Part model, mm, in its own coordinate system. A direction names the side the tool comes from. Round coordinates to 2 decimals unless told otherwise and drop trailing zeros. Loops run counter-clockwise (first coordinate to the right, second up) from the corner with the lowest first, then second, coordinate; pieces in that order, holes last.
(1) Tool access for faces 1 (the face through (30, 41, -3)), 2 (the face through (68, 13, -4)), 3 (the face through (50, 23, -3.1)), 4 (the face through (33, 12, -4)): list every direction of +Z, -Z, +X, -X, +Y, -Y with a clear straight run to the whole face (end or side of a thin tool).
(2) Cut at D-D on x = 27. List the corners of the cut face in (y, z).
(3) Mould opens along X. For faces 5 (the face through (70, 41, -3)), 6 (the face through (16.547, 5.382, 1.875)), 7 (the face through (44, 29, 3.5)) say: +X half, -X half, draft (parallel to the pull), parting line (faces both ways), or undercut.
(4) Cut at C-C on z = 1. List the corners of the cut face in (x, y) (3 decimals).
(5) Flat gauge pins, fed straight in: pin 1 (2.5 mm diameter, centred on y = 42, z = -3.5, fed in from +X); pin 2 (2.5 mm diameter, centred on y = 40, z = -3, fed in from -X); pin 3 (0.6 mm diameter, centred on x = 43.5, z = -4, fed in from -Y). Where does each tip first touch, or does it go through?
(6) Cut at A-A on y = 33.5. List the corners of the cut face in (x, z), then the cut area to 3 significant figures.
(7) Probe probe 1 along Y at (x, z) = (15, 2.7); probe 2 along Z at (x, y) = (43, 17); probe 3 along Z at (x, y) = (73.5, 20). List the from-to ranges inside material, lowest first.
(8) Cut at B-B on x = 15. List the corners of the cut face in (y, z), then the cut area to 3 significant figures.
Autodesk Inventor part; units mm, degrees
ref_plane "YZ Plane" through (0, 0, 0) normal (1, 0, 0) x (0, 1, 0)
ref_plane "XZ Plane" through (0, 0, 0) normal (0, 1, 0) x (-1, 0, 0)
ref_plane "XY Plane" through (0, 0, 0) normal (0, 0, 1) x (1, 0, 0)
sketch "Sketch1" plane through (0, 0, 0) normal (0, 0, 1) x (1, 0, 0)
  line L0 (0, 0) -> (90, 0)
  line L1 (90, 0) -> (90, 57)
  line L2 (90, 57) -> (0, 57)
  line L3 (0, 57) -> (0, 0)
  circle A0 centre (15, 53) radius 1.55
  circle A1 centre (15, 4.74) radius 1.55
  circle A2 centre (80.699, 49.825) radius 1.55
  circle A3 centre (80.699, 7.915) radius 1.55
  dimension "d0" = 57
  dimension "d1" = 90
  dimension "d2" = 3.1
  dimension "d3" = 3.1
  dimension "d4" = 3.1
  dimension "d5" = 3.1
  dimension "d6" = 4
  dimension "d7" = 15
  dimension "d8" = 48.26
  dimension "d9" = 15
  dimension "d10" = 80.699
  dimension "d11" = 7.175
  dimension "d12" = 41.91
  dimension "d13" = 80.699
extrude "Extrusion1" add sketch "Sketch1" along normal blind 3.5
sketch "Sketch2" plane through (0, 0, 0) normal (0, 0, -1) x (-1, 0, 0)
  line L0 (-70, 35) -> (-30, 35)
  line L1 (-30, 35) -> (-30, 57)
  line L2 (-30, 57) -> (-70, 57)
  line L3 (-70, 57) -> (-70, 35)
  line L4 (0, 0) -> (-90, 0)
  line L5 (-90, 57) -> (0, 57)
  line L6 (-90, 0) -> (-90, 57)
  dimension "d16" = 35
  dimension "d17" = 40
  dimension "d18" = 20
extrude "Extrusion2" add sketch "Sketch2" along normal blind 5.1
sketch "Sketch3" plane through (30, 35, 0) normal (0, -1, 0) x (1, 0, 0)
  line L0 (0, -5.1) -> (40, -5.1)
  line L1 (40, -5.1) -> (40, -3.1)
  line L2 (40, -3.1) -> (0, -3.1)
  line L3 (0, -3.1) -> (0, -5.1)
  line L4 (40, -5.1) -> (0, -5.1)
  line L5 (0, 0) -> (0, -5.1)
  line L6 (40, 0) -> (40, -5.1)
  line L7 (-30, 0) -> (60, 0)
  dimension "d21" = 3.1
extrude "Extrusion3" add sketch "Sketch3" along normal blind 25 contours L3 L2 L1 L0
chamfer "Chamfer1" distance 5 angle 45 2 edges at (70, 10, -4.1) (30, 10, -4.1)
chamfer "Chamfer2" distance 1 angle 45 2 edges at (90, 0, 1.75) (0, 0, 1.75)
chamfer "Chamfer3" distance 2 angle 45 4 edges at (13.45, 53, 0) (13.45, 4.74, 0) (79.149, 49.825, 0) (79.149, 7.915, 0)
properties part number "BeagleBoneMountingBracket"
Final values:
1. face 1: -Z, -X, +Y, -Y
1. face 2: -Z, +X, -Y
1. face 3: +X, -X, -Y
1. face 4: -Z, -X, -Y
2. outline: (0, 0) - (57, 0) - (57, 3.5) - (0, 3.5) - close
3. face 5: +X half
3. face 6: undercut
3. face 7: draft
4. outline: (0, 1) - (1, 0) - (89, 0) - (90, 1) - (90, 57) - (0, 57) - close; hole circle Ø5.1 at (15, 4.74); hole circle Ø5.1 at (15, 53); hole circle Ø5.1 at (80.699, 7.915); hole circle Ø5.1 at (80.699, 49.825)
5. pin 1: stops at x = 70
5. pin 2: stops at x = 30
5. pin 3: stops at y = 10
6. outline: (0, 0) - (90, 0) - (90, 3.5) - (0, 3.5) - close; (30, -5.1) - (70, -5.1) - (70, -3.1) - (30, -3.1) - close
6. area: 395 mm2
7. probe 1: y = 0 to 3.19, 6.29 to 51.45, 54.55 to 57
7. probe 2: z = -5.1 to -3.1, 0 to 3.5
7. probe 3: z = 0 to 3.5
8. outline: (0, 0) - (1.19, 0) - (3.19, 2) - (3.19, 3.5) - (0, 3.5) - close; (6.29, 2) - (8.29, 0) - (49.45, 0) - (51.45, 2) - (51.45, 3.5) - (6.29, 3.5) - close; (54.55, 2) - (56.55, 0) - (57, 0) - (57, 3.5) - (54.55, 3.5) - close
8. area: 170 mm2
